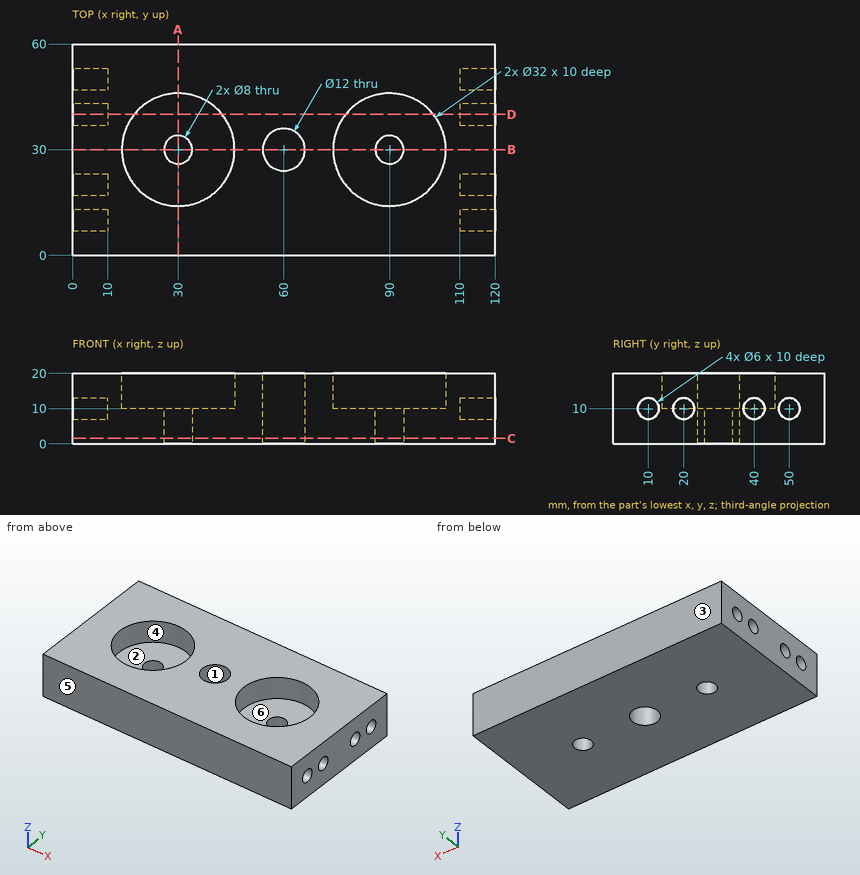
Can you work these out from the drawing? Everything is in mm from the part's minimum corner. A direction names the side the tool comes from. Coordinates: 2 decimals unless noted, no trailing zeros. Loops run counter-clockwise (first coordinate to the right, second up) from the corner with the lowest first, then second, coordinate; pieces in that order, holes last.
1) Which directions (+Z, -Z, +X, -X, +Y, -Y) give clear straight access to the entire face, cutting with the end or side of a thin tool? Please do the marked faces 1 and 2.
2) For pin 1 (3.5 mm diameter, centred on y = 40, z = 10, fed in from +X); pin 2 (3 mm diameter, centred on x = 93.5, y = 23, fed in from +Z); pin 3 (3.5 mm diameter, centred on y = 50, z = 10, fed in from -X), each with a flat end and sliding along its axis, tell me the tip position at first contact or that it passes through.
3) Thinking about a two-plate mould opening in Y: for the marked faces 3, 4, 5 and 6, which applies, pulls with the +Y half, pulls with the -Y half, needs draft (parallel to the pull), parting line crosses it, or undercut?
4) Imagine slicing it at B-B on y = 30. List the corners of the cut face in (x, z) for me, plus the area to 3 significant figures.
5) Imagine slicing it at C-C on z = 1.5. List the corners of the cut face in (x, y) for me.
6) Imagine slicing it at D-D on y = 40. List the corners of the cut face in (x, z) for me, plus the area to 3 significant figures.
7) Imagine slicing it at A-A on x = 30. List the corners of the cut face in (y, z) for me.
8) I need wall thicknesses on probe 1 along Y at (x, z) = (90, 8.25); probe 2 along Y at (x, z) = (29.5, 11.75); probe 3 along X at (y, z) = (29, 3). Which ranges of each line are inside material? Lowest first, please.
Completed:
1. face 1: +Z, -Z
1. face 2: +Z
2. pin 1: stops at x = 110
2. pin 2: stops at z = 10
2. pin 3: stops at x = 10
3. face 3: pulls with the +Y half
3. face 4: undercut
3. face 5: pulls with the -Y half
3. face 6: undercut
4. outline: (0, 0) - (26, 0) - (26, 10) - (14, 10) - (14, 20) - (0, 20) - close; (34, 0) - (54, 0) - (54, 20) - (46, 20) - (46, 10) - (34, 10) - close; (66, 0) - (86, 0) - (86, 10) - (74, 10) - (74, 20) - (66, 20) - close; (94, 0) - (120, 0) - (120, 20) - (106, 20) - (106, 10) - (94, 10) - close
4. area: 1,360 mm2
5. outline: (0, 0) - (120, 0) - (120, 60) - (0, 60) - close; hole circle Ø8 at (30, 30); hole circle Ø12 at (60, 30); hole circle Ø8 at (90, 30)
6. outline: (0, 0) - (120, 0) - (120, 7) - (110, 7) - (110, 13) - (120, 13) - (120, 20) - (102.49, 20) - (102.49, 10) - (77.51, 10) - (77.51, 20) - (42.49, 20) - (42.49, 10) - (17.51, 10) - (17.51, 20) - (0, 20) - (0, 13) - (10, 13) - (10, 7) - (0, 7) - close
6. area: 1,780 mm2
7. outline: (0, 0) - (26, 0) - (26, 10) - (14, 10) - (14, 20) - (0, 20) - close; (34, 0) - (60, 0) - (60, 20) - (46, 20) - (46, 10) - (34, 10) - close
8. probe 1: y = 0 to 26, 34 to 60
8. probe 2: y = 0 to 14.01, 45.99 to 60
8. probe 3: x = 0 to 26.13, 33.87 to 54.08, 65.92 to 86.13, 93.87 to 120
